Build history of the part. All positions in model axes, mm. A direction names the side the tool comes from. Coordinates: 2 decimals unless noted, no trailing zeros. Write each loop counter-clockwise with the first axis right and the second up, starting at its lowest first coordinate (ties: lowest second). Pieces come first, ordered by that corner, then holes.
Autodesk Inventor part; units mm, degrees
ref_plane "YZ Plane" through (0, 0, 0) normal (1, 0, 0) x (0, 1, 0)
ref_plane "XZ Plane" through (0, 0, 0) normal (0, 1, 0) x (-1, 0, 0)
ref_plane "XY Plane" through (0, 0, 0) normal (0, 0, 1) x (1, 0, 0)
sketch "Náčrt1" plane through (0, 0, 0) normal (0, 1, 0) x (-1, 0, 0)
  line L0 (0, 0) -> (7.0755, 0)
  line L1 (6.7377, 13.35) -> (6.7377, -13.35)
  line L2 (4.2782, 13.5) -> (4.2782, -13.5)
  line L3 (3.5377, 9.35) -> (3.5377, -9.35)
  circle A0 centre (6.7377, -13.35) radius 1.7
  line L4 (3.5377, -9.35) -> (1.5377, -9.35)
  line L5 (1.5377, -9.35) -> (1.5377, -16.55)
  line L6 (1.5377, -16.55) -> (3.5377, -16.55)
  line L7 (3.5377, -16.55) -> (3.5377, -9.35)
  arc A1 (6.7377, -16.55) -> (6.7377, -10.15) centre (6.7377, -13.35) ccw
  line L8 (6.7377, -10.15) -> (3.5377, -10.15)
  line L9 (6.7377, -16.55) -> (1.5377, -16.55)
  line L10 (0.3377, -9.35) -> (-1.6623, -9.35)
  line L11 (-1.6623, -9.35) -> (-1.6623, -16.55)
  line L12 (-1.6623, -16.55) -> (0.3377, -16.55)
  line L13 (0.3377, -16.55) -> (0.3377, -9.35)
  line L14 (-1.6623, -16.55) -> (-1.6623, -16.55)
  line L15 (-1.6623, -16.55) -> (1.5377, -16.55)
  line L16 (1.5377, -9.35) -> (0.3377, -9.35)
  line L17 (-0.6623, -10.15) -> (3.5377, -10.15)
  line L18 (3.5377, -10.15) -> (3.5377, 0)
  line L19 (3.5377, 0) -> (-0.6623, 0)
  line L20 (-0.6623, 0) -> (-0.6623, -10.15)
  point P0 (2.5377, 0)
  point P1 (3.5377, -10.15)
  point P2 (2.5377, -9.35)
  point P3 (1.5377, -10.15)
  point P4 (3.5377, -9.35)
  point P5 (-0.6623, -9.35)
  point P6 (3.5377, 0)
  point P7 (3.5377, 0)
  dimension "d0" = 26.7
  dimension "d1" = 27
  dimension "d2" = 18.7
  dimension "d4" = 3.4
  dimension "d5" = 2
  dimension "d7" = 1.5
  dimension "d9" = 2
  dimension "d11" = 1.2
  dimension "d19" = 1
extrude "Vysunutí1" add sketch "Náčrt1" along normal blind 1 contours L0 L3 L4 L16 L10 L20 L19 | L7 L17 L5 L4 | L10 L13 L17 L20 | L8 A1 L9 L7 | L5 L17 L13 L16 | L5 L15 L13 L17
extrude "Vysunutí2" add sketch "Náčrt1" along normal blind 4 contours L7 L17 L5 L4 | L20 L17 L13 L12 L11 L10 | L10 L13 L17 L20 | L7 L6 L5 L17
fillet "Zaoblení1" radius 3 1 edges at (0.6623, 0.5, -9.35)
fillet "Zaoblení4" radius 3 1 edges at (-3.5377, 0.5, -10.15)
mirror "Zrcadlit2" about plane through (-3.5377, 0, 0) normal (0, 0, 1) of "Vysunutí1", "Vysunutí2", "Zaoblení1", "Zaoblení4"
properties part number "esp holder"
(1) Two-plate mould, pull along X, no slides. Class faces 5 (the flat face through (1.662, 2, -13)), 6 (the flat face through (-0.338, 2, 13)), 7 (the flat face through (-3, 2, -9.35)): pulls with the +X half, pulls with the -X half, needs draft (parallel to the pull), parting line crosses it, or undercut.
(2) Flat gauge pins, fed straight in: P1, Ø0.8, axis at y = 0.5, z = 3.5, coming from the +X side; P2, Ø1.1, axis at y = 0.5, z = -2.5, coming from the -X side; P3, Ø3, axis at x = -6.74, z = -13.35, coming from the +Y side. Where does each tip first touch, or does it go through?
(3) 3-axis set-ups, long thin cutter, end or side, ignore diameter. For faces 1 (the cylindrical face through (0.93, 0.51, -8.35)), 2 (the cylindrical face through (-4.44, 0.493, -9.295)), 3 (the flat face through (1, 2, -9.35)), 4 (the flat face through (-0.338, 2, -13)): which of +Z, -Z, +X, -X, +Y, -Y reach the whole face in a straight line?
(4) Slice it at A-A, the plane z = 13.35. List the corners of the cut face in (x, y).
(5) Slice it at D-D, the plane x = -4.5. List the corners of the cut face in (y, z), and give its area (3 significant figures).
(6) Slice it at B-B, the plane x = -6. List the corners of the cut face in (y, z), and give its area (3 significant figures).
(7) Probe L1, parallel to X at y = 0.55, z = 13.35; L2, parallel to X at y = 3.65, z = -13.5; L3, parallel to Z at x = -2, y = 3.35. List the from-to ranges inside material, lowest first.
(8) Slice it at C-C, the plane x = -3. List the corners of the cut face in (y, z), and give its area (3 significant figures).
Results:
1. face 5: pulls with the +X half
1. face 6: undercut
1. face 7: needs draft
2. P1: stops at x = 0.66
2. P2: stops at x = -3.54
2. P3: passes through
3. face 1: +X, +Y, -Y
3. face 2: -X, +Y, -Y
3. face 3: +X, -X, +Y
3. face 4: +Z, -Z, +Y
4. outline: (-9.94, 0) - (-8.44, 0) - (-8.44, 1) - (-9.94, 1) - close; (-5.04, 0) - (1.66, 0) - (1.66, 4) - (-0.34, 4) - (-0.34, 1) - (-1.54, 1) - (-1.54, 4) - (-3.54, 4) - (-3.54, 1) - (-5.04, 1) - close
5. outline: (0, -16.55) - (1, -16.55) - (1, -9.35) - (0, -9.35) - close; (0, 9.35) - (1, 9.35) - (1, 16.55) - (0, 16.55) - close
5. area: 14.4 mm2
6. outline: (0, -16.55) - (1, -16.55) - (1, -14.88) - (0, -14.88) - close; (0, -11.82) - (1, -11.82) - (1, -10.1) - (0, -10.1) - close; (0, 10.1) - (1, 10.1) - (1, 11.82) - (0, 11.82) - close; (0, 14.88) - (1, 14.88) - (1, 16.55) - (0, 16.55) - close
6. area: 6.77 mm2
7. L1: x = -9.94 to -8.44, -5.04 to 1.66
7. L2: x = -3.54 to -1.54, -0.34 to 1.66
7. L3: z = -16.55 to -9.35, 9.35 to 16.55
8. outline: (0, -16.55) - (4, -16.55) - (4, -9.35) - (1, -9.35) - (1, 9.35) - (4, 9.35) - (4, 16.55) - (0, 16.55) - close
8. area: 76.3 mm2
